For this review, take the finished solid that the model builds, in its own axes (mm). A direction names the side the tool comes from. Coordinates: 2 decimals unless noted, no trailing zeros. Loops run counter-clockwise (first coordinate to the right, second up) from the corner with the lowest first, then second, coordinate; pieces in that order, holes last. Notation, with made-up numbers: M 53,45.5 L 91,45.5 A18 cw 91,70.5 Z; hole C 32,-12 d8. An arc over 180 degrees is marked long. Answer as a JSON object with one key per item and string values. Group by question number.
Item 1: Mouldability with a two-part tool opening along X and no side actions: class faces 1 (the face through (-21, 107, 48)), 2 (the face through (-40, 205, 51)), 3 (the face through (-12.01, 1.48, 61.09)) as +X half, -X half, draft (parallel to the pull), parting line (faces both ways), or undercut.
Item 2: Insertion check: pin 1 (6 mm diameter, centred on x = -17.5, y = 207.5, fed in from -Z); pin 2 (1.5 mm diameter, centred on y = 214, z = 22.5, fed in from -X); pin 3 (7 mm diameter, centred on x = -30, y = 107.5, fed in from +Z). Each pin has a flat end and moves straight along its axis. Give the tip position at first contact, or say it passes through.
Item 3: Add section B-B (x = -5). State the section outline as (y, z) points, then the cut area to 3 significant figures.
Item 4: Tool access review of faces 4 (the face through (-12, 3, 24)), 5 (the face through (-21, 108, 53)), 6 (the face through (-13.99, 213.52, 61.09)): name each direction out of +Z, -Z, +X, -X, +Y, -Y from which nothing blocks a thin tool from reaching the whole face with its end or side.
Item 5: Add section A-A (x = -30). State the section outline as (y, z) points.
Item 6: Add section D-D (z = 63). State the section outline as (x, y) points, then the cut area to 3 significant figures.
Item 7: Add section C-C (y = 107.5). State the section outline as (x, z) points.
Item 8: Wall thickness on L1, parallel to Y at x = -30, z = 51; L2, parallel to Z at x = -13, y = 213.7; L3, parallel to Y at x = -18, z = 69.5: over which ranges is each line inside the solid? List them lowest first. Write a range as from..to.
Autodesk Fusion 360 part; units mm, degrees
sketch "스케치1" plane through (0, 0, 0) normal (0, 1, 0) x (1, 0, 0)
  line L0 (0, 0) -> (0, -105)
  line L1 (0, 0) -> (-3, 0)
  line L2 (-3, 0) -> (-3, -102)
  line L3 (-3, -102) -> (-20, -102)
  line L4 (0, -105) -> (-20, -105)
  line L5 (-20, -105) -> (-20, -102)
  dimension "d1" = 105
  dimension "d2" = 3
  dimension "d3" = 102
  dimension "d4" = 17
extrude "돌출1" add sketch "스케치1" along normal blind 215
sketch "스케치2" plane through (0, 0, 0) normal (0, -1, 0) x (1, 0, 0)
  line L0 (-3, 0) -> (0, 0)
  line L1 (0, 0) -> (0, 105)
  line L2 (0, 105) -> (-20, 105)
  line L3 (-20, 105) -> (-20, 102)
  line L4 (-20, 102) -> (-3, 102)
  line L5 (-3, 102) -> (-3, 0)
  line L6 (0, 105) -> (-20, 105)
  line L7 (-20, 105) -> (-20, 0)
  line L8 (-20, 0) -> (0, 0)
  line L9 (0, 0) -> (0, 105)
  line L10 (-3, 102) -> (-3, 73)
  line L11 (-3, 73) -> (-20, 73)
  line L12 (-20, 73) -> (-20, 53)
  line L13 (-20, 53) -> (-3, 53)
  line L14 (-3, 53) -> (-3, 73)
  line L15 (-20, 53) -> (-13, 53)
  line L16 (-13, 53) -> (-13, 63)
  line L17 (-13, 63) -> (-20, 63)
  line L18 (-20, 63) -> (-20, 53)
  circle A0 centre (-13, 63) radius 2.15
  dimension "d11" = 29
  dimension "d12" = 17
  dimension "d13" = 20
  dimension "d14" = 7
  dimension "d15" = 10
  dimension "d16" = 4.3
extrude "돌출2" add sketch "스케치2" against normal blind 3 contours L0 L1 L2 L3 L4 L5 L6 L7 L8 L9 L10 L14 | L5 L7 L8 L13 L15 | L5 L7 L11 L12 L13 L14 L16 L17 A0 | L4 L5 L7 L10 L11 | L7 L12 L13 L15 L16 L17 L18 A0
sketch "스케치3" plane through (0, 215, 0) normal (0, 1, 0) x (-1, 0, 0)
  line L0 (0, 0) -> (3, 0)
  line L1 (3, 0) -> (3, 102)
  line L2 (3, 102) -> (20, 102)
  line L3 (20, 102) -> (20, 105)
  line L4 (20, 105) -> (0, 105)
  line L5 (0, 105) -> (0, 0)
  line L6 (0, 105) -> (20, 105)
  line L7 (20, 105) -> (20, 0)
  line L8 (20, 0) -> (0, 0)
  line L9 (0, 0) -> (0, 105)
  line L10 (3, 102) -> (3, 73)
  line L11 (3, 73) -> (20, 73)
  line L12 (20, 73) -> (20, 53)
  line L13 (20, 53) -> (3, 53)
  line L14 (3, 53) -> (3, 73)
  line L15 (20, 53) -> (13, 53)
  line L16 (13, 53) -> (13, 63)
  line L17 (13, 63) -> (20, 63)
  line L18 (20, 63) -> (20, 53)
  circle A0 centre (13, 63) radius 2.15
  dimension "d17" = 29
  dimension "d18" = 17
  dimension "d19" = 20
  dimension "d20" = 7
  dimension "d21" = 10
  dimension "d22" = 4.3
extrude "돌출3" add sketch "스케치3" against normal blind 3 contours L1 L7 L8 L13 L15 | L1 L7 L11 L12 L13 L14 L16 L17 A0 | L1 L2 L7 L10 L11 | L7 L12 L13 L15 L16 L17 L18 A0
sketch "스케치4" plane through (-3, 0, 0) normal (-1, 0, 0) x (0, -1, 0)
  line L0 (-212, 102) -> (-212, 0)
  line L1 (-212, 0) -> (-3, 0)
  line L2 (-3, 0) -> (-3, 102)
  line L3 (-3, 102) -> (-212, 102)
  line L4 (-212, 102) -> (-212, 53)
  line L5 (-212, 53) -> (-195, 53)
  line L6 (-195, 53) -> (-195, 48)
  line L7 (-195, 48) -> (-212, 48)
  line L8 (-212, 48) -> (-212, 53)
  line L9 (-3, 53) -> (-20, 53)
  line L10 (-20, 53) -> (-20, 48)
  line L11 (-20, 48) -> (-3, 48)
  line L12 (-3, 48) -> (-3, 53)
  line L13 (-195, 53) -> (-112.5, 53)
  line L14 (-112.5, 53) -> (-102.5, 53)
  line L15 (-102.5, 53) -> (-102.5, 48)
  line L16 (-102.5, 48) -> (-112.5, 48)
  line L17 (-112.5, 48) -> (-112.5, 53)
  dimension "d23" = 49
  dimension "d24" = 17
  dimension "d25" = 5
  dimension "d26" = 17
  dimension "d27" = 5
  dimension "d28" = 82.5
  dimension "d29" = 10
  dimension "d30" = 5
extrude "돌출4" add sketch "스케치4" along normal blind 37 contours L14 L15 L16 L17 | L0 L5 L6 L7 L8 | L2 L9 L10 L11 L12
extrude "돌출5" add 1 faces at (-26.6667, 3, 49.6667) along direction (0, -1, 0) blind 3
extrude "돌출6" add 1 faces at (-33.3333, 212, 51.3333) along direction (0, 1, 0) blind 3
sketch "스케치5" plane through (0, 0, 53) normal (0, 0, 1) x (-1, 0, 0)
  line L0 (3, -102.5) -> (3, -112.5)
  line L1 (3, -112.5) -> (40, -112.5)
  line L2 (40, -112.5) -> (40, -102.5)
  line L3 (40, -102.5) -> (3, -102.5)
  line L4 (40, -102.5) -> (20, -102.5)
  line L5 (20, -102.5) -> (20, -112.5)
  line L6 (20, -112.5) -> (40, -112.5)
  line L7 (40, -112.5) -> (40, -102.5)
  circle A0 centre (30, -107.5) radius 2.65
  circle A1 centre (30, -205) radius 2.65
  circle A2 centre (30, -10) radius 2.65
  dimension "d37" = 20
  dimension "d43" = 5.3
  dimension "d49" = 5.3
  dimension "d50" = 5.3
extrude "돌출7" cut sketch "스케치5" against normal blind 5 contours A0 | A1 | A2
fillet "필렛1" radius 2.5 1 edges at (0, 107.5, 105)
From the geometry:
{
 "1": {"face 1": "draft", "face 2": "-X half", "face 3": "undercut"},
 "2": {"pin 1": "stops at z = 48", "pin 2": "stops at x = -20", "pin 3": "stops at z = 53"},
 "3": {"outline": "M 0,0 L 3,0 L 3,48 L 20,48 L 20,53 L 3,53 L 3,102 L 212,102 L 212,53 L 195,53 L 195,48 L 212,48 L 212,0 L 215,0 L 215,105 L 0,105 Z; M 102.5,48 L 112.5,48 L 112.5,53 L 102.5,53 Z", "area": "1,480 mm²"},
 "4": {"face 4": "-Z, -X", "face 5": "-X", "face 6": "+Y, -Y"},
 "5": {"outline": "M 0,48 L 7.35,48 L 7.35,53 L 0,53 Z; M 12.65,48 L 20,48 L 20,53 L 12.65,53 Z; M 102.5,48 L 104.85,48 L 104.85,53 L 102.5,53 Z; M 110.15,48 L 112.5,48 L 112.5,53 L 110.15,53 Z; M 195,48 L 202.35,48 L 202.35,53 L 195,53 Z; M 207.65,48 L 215,48 L 215,53 L 207.65,53 Z"},
 "6": {"outline": "M -20,0 L -15.15,0 L -15.15,3 L -20,3 Z; M -20,212 L -15.15,212 L -15.15,215 L -20,215 Z; M -10.85,0 L 0,0 L 0,215 L -10.85,215 L -10.85,212 L -3,212 L -3,3 L -10.85,3 Z", "area": "721 mm²"},
 "7": {"outline": "M -40,48 L -32.65,48 L -32.65,53 L -40,53 Z; M -27.35,48 L -3,48 L -3,0 L 0,0 L 0,102.5 A2.5 ccw -2.5,105 L -20,105 L -20,102 L -3,102 L -3,53 L -27.35,53 Z"},
 "8": {"L1": "y = 0..7.35, 12.65..20, 102.5..104.85, 110.15..112.5, 195..202.35, 207.65..215", "L2": "z = 0..60.85, 65.15..105", "L3": "y = 0..3, 212..215"}
}
